Could you check a few things on this model? Use its own coordinates, in mm. A direction names the side the tool comes from. Give positions to 0.01 mm unless a question says otherwise; leave off trailing zeros. Loops run counter-clockwise (first coordinate to the right, second up) from the corner with the lowest first, then second, coordinate; pieces in that order, holes last. Notation, with made-up numbers: M 56.25,35.5 L 70.25,35.5 A28 cw 70.25,67.5 Z; hole C 89,-10 d2. An arc over 180 degrees is marked long. Answer in a Markdown table with one row per item. Add a question column.
1. If we section it at B-B on z = -9: List the corners of the cut face in (x, y) for me, then the cut area to 3 significant figures.
2. If we section it at D-D on z = -2.25: List the corners of the cut face in (x, y) for me, then the cut area to 3 significant figures.
3. Thinking about a two-plate mould opening in Z: for faces 3 (the cylindrical face through (1.521, 9.352, -7.526)), 4 (the cylindrical face through (20, 2, -9)), 5 (the flat face through (3, 17, -9)), which applies, released by +Z, released by -Z, zero draft, split by the parting line, or undercut?
4. I need wall thicknesses on line 1 along Y through (x, z) = (1.45, -9); line 2 along X through (y, z) = (1.6, -9); line 3 along X through (y, z) = (23, -10). Which ranges of each line are inside material? Lowest first, please. Write a range as from..to.
5. Which directions (+Z, -Z, +X, -X, +Y, -Y) give clear straight access to the entire face, cutting with the end or side of a thin tool? Please do faces 1 (the flat face through (17, 3, -7)), 2 (the flat face through (32, 1, -9)).
6. I'm going to push flat-ended pins straight in: pin 1 Ø5.5 at (x, z) = (23, -10.5) entering from +Y; pin 2 Ø10 at (y, z) = (28.5, -9.5) entering from +X; pin 3 Ø5 at (x, y) = (22, 6) entering from -Z. Where does each tip first touch, or does it pass through?
7. If we section it at A-A on x = 18: List the corners of the cut face in (y, z) for me, then the cut area to 3 significant figures.
```python
from build123d import *

# Parameters (mm, degrees)
SKETCH1_W           = 32
SKETCH1_H           = 18
BOSS_EXTRUDE1_DEPTH = 3
SKETCH2_W           = 3
SKETCH2_H           = 18
BOSS_EXTRUDE2_DEPTH = 29
SKETCH3_R           = 2
CUT_EXTRUDE1_DEPTH  = 47.786750261
SKETCH4_R           = 2
CUT_EXTRUDE2_DEPTH  = 47.786750261


with BuildPart() as part:
    # Sketch1 → Boss-Extrude1 (new body)
    with BuildSketch(Plane(origin=(0, 0, 0), x_dir=(1, 0, 0), z_dir=(0, 1, 0))):
        with Locations((16, 9)):
            Rectangle(SKETCH1_W, SKETCH1_H)
    extrude(amount=BOSS_EXTRUDE1_DEPTH)

    # Sketch2 → Boss-Extrude2 (add)
    with BuildSketch(Plane(origin=(0, 3, 0), x_dir=(1, 0, 0), z_dir=(0, 1, 0))):
        with Locations((1.5, 9)):
            Rectangle(SKETCH2_W, SKETCH2_H)
    extrude(amount=BOSS_EXTRUDE2_DEPTH)

    # Sketch3 → Cut-Extrude1 (cut, through all)
    with BuildSketch(Plane(origin=(0, 3, 0), x_dir=(1, 0, 0), z_dir=(0, 1, 0))):
        with Locations(Location((18, 9, 0), (0, 0, 270))):
            Circle(SKETCH3_R)
    extrude(amount=-CUT_EXTRUDE1_DEPTH, mode=Mode.SUBTRACT)

    # Sketch4 → Cut-Extrude2 (cut, through all)
    with BuildSketch(Plane(origin=(3, 0, 0), x_dir=(0, 0, -1), z_dir=(1, 0, 0))):
        with Locations((9, 20)):
            Circle(SKETCH4_R)
        with Locations((9, 8)):
            Circle(SKETCH4_R)
    extrude(amount=-CUT_EXTRUDE2_DEPTH, mode=Mode.SUBTRACT)


solid = part.part
```
Results:
| question | item | result |
|---|---|---|
| 1 | outline | M 0,0 L 16,0 L 16,3 L 3,3 L 3,6 L 0,6 Z; M 0,10 L 3,10 L 3,18 L 0,18 Z; M 0,22 L 3,22 L 3,32 L 0,32 Z; M 20,0 L 32,0 L 32,3 L 20,3 Z |
| 1 | area | 147 mm2 |
| 2 | outline | M 0,0 L 32,0 L 32,3 L 3,3 L 3,32 L 0,32 Z |
| 2 | area | 183 mm2 |
| 3 | face 3 | undercut |
| 3 | face 4 | undercut |
| 3 | face 5 | zero draft |
| 4 | line 1 | 0..6, 10..18, 22..32 |
| 4 | line 2 | 0..16, 20..32 |
| 4 | line 3 | 0..3 |
| 5 | face 1 | +Z, -Z, +X, +Y |
| 5 | face 2 | +Z, -Z, +X, +Y, -Y |
| 6 | pin 1 | y = 3 |
| 6 | pin 2 | x = 3 |
| 6 | pin 3 | through |
| 7 | outline | M 0,-18 L 3,-18 L 3,-11 L 0,-11 Z; M 0,-7 L 3,-7 L 3,0 L 0,0 Z |
| 7 | area | 42.0 mm2 |
